Verification items for this drawing (mm, ordinates from the low corner). Round coordinates to 2 decimals unless told otherwise and drop trailing zeros. Loops run counter-clockwise (first coordinate to the right, second up) from the corner with the lowest first, then second, coordinate; pieces in that order, holes last. Notation, with made-up numbers: M 26,62.25 L 70,62.25 A14 ccw 70,83.25 Z; hole C 79.25,88.5 d3. An arc over 180 degrees is marked long. Write item = value, one per line. Start each with the question number.
(1) Cross-section at B-B on x = 6.5. Record the boundary of the cut face in (y, z), plus the area to 3 significant figures.
(2) Cross-section at C-C on y = 42. Record the boundary of the cut face in (x, z).
(3) Scan lines: L1, parallel to Y at x = 16, z = 10; L2, parallel to Y at x = 18.75, z = 7.75; L3, parallel to Z at x = 9.75, y = 178. Record each from-to range of solid material in increasing order. Write a range as from..to.
(4) Go/stop test with flat-tipped pins: P1, Ø8.5, axis at y = 12, z = 10, coming from the -X side; P2, Ø1, axis at x = 4.5, y = 185, coming from the -Z side; P3, Ø6, axis at x = 4, y = 144.5, coming from the -Z side; P4, Ø1.5, axis at x = 16.5, y = 203, coming from the +Z side. Record where each tip stops, or that it passes through.
(5) Cross-section at A-A on z = 10. Record the boundary of the cut face in (x, y), plus the area to 3 significant figures.
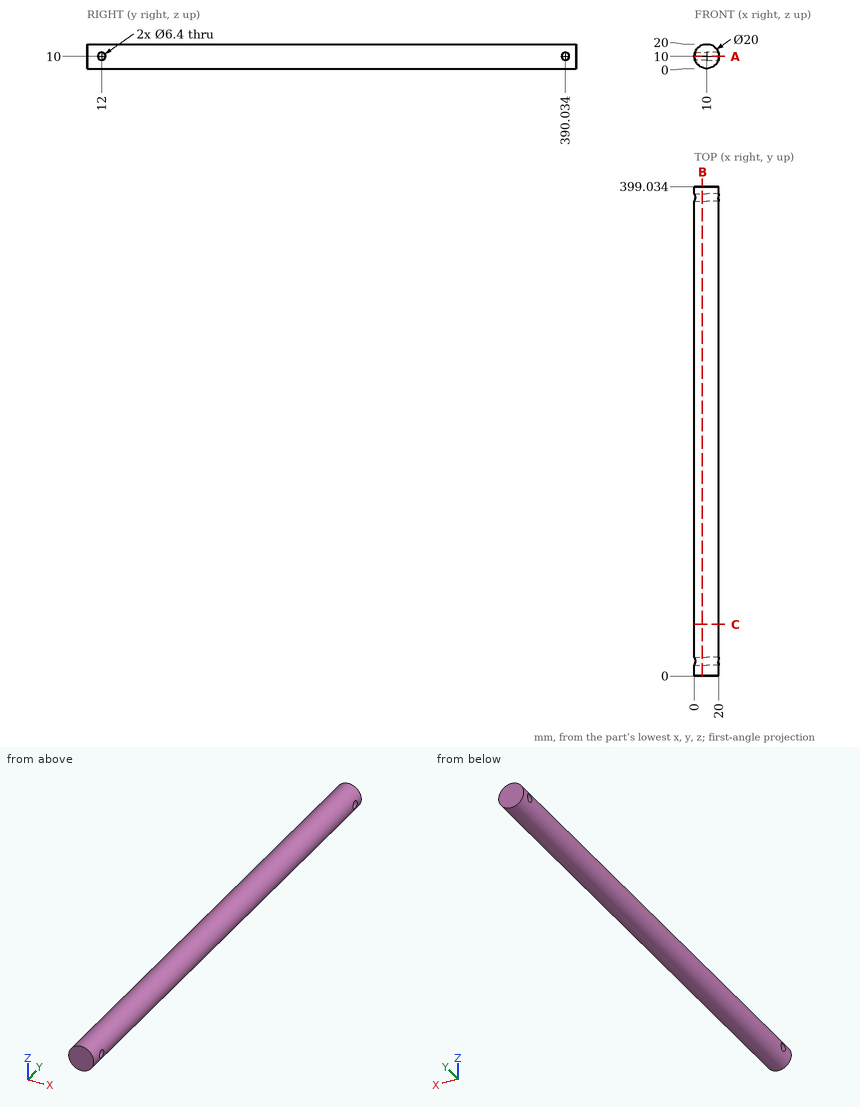
Result:
q1.outline = M 0,0.63 L 399.03,0.63 L 399.03,19.37 L 0,19.37 Z; hole C 12,10 d6.4; hole C 390.03,10 d6.4
q1.area = 7,410 mm^2
q2.outline = C 10,10 d20
q3.L1 = 0..8.8, 15.2..386.83, 393.23..399.03
q3.L2 = 0..9.72, 14.28..387.76, 392.31..399.03
q3.L3 = 0..20
q4.P1 = 0
q4.P2 = 1.34
q4.P3 = 0.46
q4.P4 = 18.18
q5.outline = M 0,0 L 20,0 L 20,8.8 L 0,8.8 Z; M 0,15.2 L 20,15.2 L 20,386.83 L 0,386.83 Z; M 0,393.23 L 20,393.23 L 20,399.03 L 0,399.03 Z
q5.area = 7,720 mm^2
